```python
from build123d import *

# Parameters (mm, degrees)
SKETCH_1_R             = 2.5
SKETCH_1_R_2           = 1
EXTRUDE_1_DEPTH        = 2.3
SKETCH_1_3_R           = 3.05
SKETCH_1_3_R_2         = 2.5
EXTRUDE_2_DEPTH        = 0.6
CHAMFER_1_SIZE         = 0.2
CHAMFER_1_SIZE2        = 0.115470054
CHAMFER_1_PART_2_SIZE  = 0.2
CHAMFER_1_PART_2_SIZE2 = 0.115470054


with BuildPart() as part:
    # Sketch 1 → Extrude 1 (new body)
    with BuildSketch(Plane(origin=(0, 0, 0), x_dir=(1, 0, 0), z_dir=(0, 1, 0))):
        Circle(SKETCH_1_R)
        Circle(SKETCH_1_R_2, mode=Mode.SUBTRACT)
    extrude(amount=EXTRUDE_1_DEPTH)

    # Sketch 1_3 → Extrude 2 (add)
    with BuildSketch(Plane(origin=(0, 0, 0), x_dir=(1, 0, 0), z_dir=(0, 1, 0))):
        Circle(SKETCH_1_3_R)
        Circle(SKETCH_1_3_R_2, mode=Mode.SUBTRACT)
    extrude(amount=EXTRUDE_2_DEPTH)

    # Chamfer 1
    chamfer_1_edges = [part.edges().sort_by_distance(p)[0] for p in [
        (-2.5, 2.3, 0),
    ]]
    chamfer_1_side = [part.faces().sort_by_distance(p)[0] for p in [
        (-2.5, 1.45, 0),
    ]]
    chamfer(chamfer_1_edges, length=CHAMFER_1_SIZE, length2=CHAMFER_1_SIZE2, reference=chamfer_1_side[0])

    # Chamfer 1 part 2
    chamfer_1_part_2_edges = [part.edges().sort_by_distance(p)[0] for p in [
        (-3.05, 0, 0),
    ]]
    chamfer_1_part_2_side = [part.faces().sort_by_distance(p)[0] for p in [
        (-2.963732973, 0, 0),
    ]]
    chamfer(chamfer_1_part_2_edges, length=CHAMFER_1_PART_2_SIZE, length2=CHAMFER_1_PART_2_SIZE2, reference=chamfer_1_part_2_side[0])


solid = part.part
```
Can you work these out from the model? Positions are in its coordinate system, mm. Coordinates: 2 decimals unless noted, no trailing zeros. Order: outer loops, then holes, each group sorted by start corner. A loop starts at its lowest first (then second) coordinate and runs counter-clockwise, first axis right, second up.
1. Thinking about a two-plate mould opening in Z: for faces 1 (the face through (0, 1, 1)), 2 (the face through (1.2, 0, 0)), 3 (the face through (-0.54, 1.34, 2.44)), which applies, +Z half, -Z half, draft (parallel to the pull), parting line (faces both ways), or undercut?
2. I need wall thicknesses on line 1 (X direction, y = 1.85, z = 0); line 2 (Y direction, x = -2.5, z = 1); line 3 (Z direction, x = 0, y = 0.55). Which ranges of each line are inside material? Lowest first, please.
3. If we section it at A-A (x = 0): Please give me the cut outline in (y, z), then the cut area to 3 significant figures.
4. If we section it at C-C (y = 1.2): Please give me the cut outline in (x, z).
5. If we section it at B-B (z = 0): Please give me the cut outline in (x, y), then the cut area to 3 significant figures.
6. If we section it at D-D (y = 0.2): Please give me the cut outline in (x, z), then the cut area to 3 significant figures.
Entries:
1. face 1: undercut
1. face 2: draft
1. face 3: parting line
2. line 1: x = -2.5 to -1, 1 to 2.5
2. line 2: y = 0 to 0.6
2. line 3: z = -3.05 to -1, 1 to 3.05
3. outline: (0, -2.85) - (0.12, -3.05) - (0.6, -3.05) - (0.6, -2.5) - (2.1, -2.5) - (2.3, -2.38) - (2.3, -1) - (0, -1) - close; (0, 1) - (2.3, 1) - (2.3, 2.38) - (2.1, 2.5) - (0.6, 2.5) - (0.6, 3.05) - (0.12, 3.05) - (0, 2.85) - close
3. area: 7.51 mm2
4. outline: circle Ø5 at (0, 0); hole circle Ø2 at (0, 0)
5. outline: (-3.05, 0.12) - (-2.85, 0) - (-1, 0) - (-1, 2.3) - (-2.38, 2.3) - (-2.5, 2.1) - (-2.5, 0.6) - (-3.05, 0.6) - close; (1, 0) - (2.85, 0) - (3.05, 0.12) - (3.05, 0.6) - (2.5, 0.6) - (2.5, 2.1) - (2.38, 2.3) - (1, 2.3) - close
5. area: 7.51 mm2
6. outline: circle Ø6.1 at (0, 0); hole circle Ø2 at (0, 0)
6. area: 26.1 mm2
